Verification items for the finished model (mm, model axes). Face numbers are marked on the shaded views. Coordinates: 2 decimals unless noted, no trailing zeros. Order: outer loops, then holes, each group sorted by start corner. A loop starts at its lowest first (then second) coordinate and runs counter-clockwise, first axis right, second up. Notation, with made-up numbers: M 78,-35.5 L 92,-35.5 A14 cw 92,-30.5 Z; hole C 40,62.25 d7. An arc over 180 degrees is marked long. Answer as a JSON object with one key per item and string values. Group by question number.
(1) Gauge pin test, flat ends, axial feed: pin 1 Ø1 at (y, z) = (29, 10) entering from +X; pin 2 Ø4 at (y, z) = (17, 13.5) entering from +X; pin 3 Ø1.5 at (y, z) = (36.5, 12.5) entering from +X. Record the tip position at first contact, or that the pin passes through.
(2) Cross-section at A-A (x = 18). Enter the section's corners in (y, z).
(3) Material ranges on line 1 (X direction, y = 33.75, z = 8.5); line 2 (X direction, y = 16, z = 10); line 3 (X direction, y = 27, z = 11.5), recorded low to high.
(4) Cross-section at B-B (y = 24.75). Enter the section's corners in (x, z), plus the area to 3 significant figures.
(5) Cross-section at C-C (z = 10). Enter the section's corners in (x, y).
(6) Cross-section at D-D (x = -55.5). Enter the section's corners in (y, z).
(7) Mould release check, pull along Y, two halves, no side actions. Record for the marked faces 1, 2, 3 and 4: released by +Y, released by -Y, zero draft, split by the parting line, or undercut.
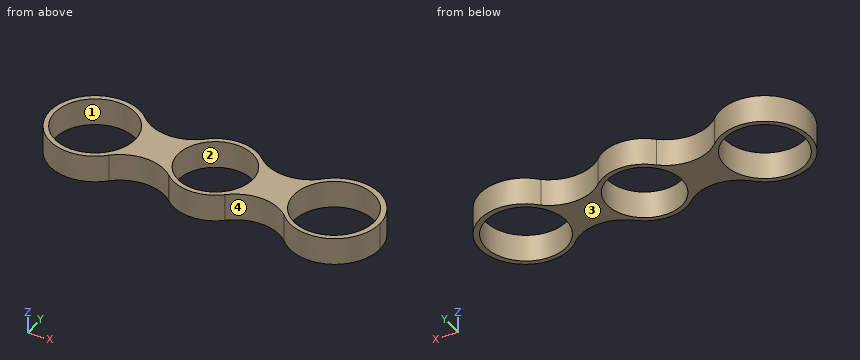
from build123d import *

# Parameters (mm, degrees)
F1_DEPTH = 8
F3_DEPTH = 8
F4_D     = 23.6
F5_D     = 22


# Not quite as in the source:
# - a feature names something its author has since deleted; it is built from what else it names


with BuildPart() as f1:
    # F0 (on Top) → F1 (new body)
    with BuildSketch(Plane.XY):
        with BuildLine():
            ThreePointArc((30.2364596242, 25.5677551031), (18.556965651, 37.3204786398), (6.7314716859, 25.7146705041))
            ThreePointArc((6.7314716859, 25.7146705041), (18.4100473802, 13.8150315665), (30.2364596242, 25.5677551031))
        make_face()
    extrude(amount=F1_DEPTH)

    # F2 (on face) → F3 (join)
    with BuildSketch(Plane.XY.offset(8)):
        with BuildLine():
            ThreePointArc((-42.5114348153, 35.1915450581), (-65.2620832709, 26.0556201481), (-42.5726949965, 16.7685975444))
            ThreePointArc((-42.5726949965, 16.7685975444), (-39.7847972392, 21.021355147), (-38.8073447634, 26.0116364807))
            ThreePointArc((-38.8073447634, 26.0116364807), (-39.7682713179, 30.9611567757), (-42.5114348153, 35.1915450581))
        make_face()
        with BuildLine():
            ThreePointArc((-38.8073447634, 26.0116364807), (-39.7847972392, 21.021355147), (-42.5726949965, 16.7685975444))
            ThreePointArc((-42.5726949965, 16.7685975444), (-33.87370444, 20.218317429), (-25.1016516698, 16.9588551759))
            ThreePointArc((-25.1016516698, 16.9588551759), (-29.0338445102, 25.8480071098), (-25.3315074449, 34.8353238892))
            ThreePointArc((-25.3315074449, 34.8353238892), (-33.9883630197, 31.7873549926), (-42.5114348153, 35.1915450581))
            ThreePointArc((-42.5114348153, 35.1915450581), (-39.7682713179, 30.9611567757), (-38.8073447634, 26.0116364807))
        make_face()
        with BuildLine():
            ThreePointArc((-24.8354704192, 16.7176675443), (-24.9677312973, 16.8391770918), (-25.1016516698, 16.9588551759))
            ThreePointArc((-25.1016516698, 16.9588551759), (-24.9694362403, 16.8372954701), (-24.8354704192, 16.7176675443))
        make_face()
        with BuildLine():
            ThreePointArc((-25.3315074449, 34.8353238892), (-29.0338445102, 25.8480071098), (-25.1016516698, 16.9588551759))
            ThreePointArc((-25.1016516698, 16.9588551759), (-24.9677312973, 16.8391770918), (-24.8354704192, 16.7176675443))
            ThreePointArc((-24.8354704192, 16.7176675443), (-16.6524528686, 13.6328843719), (-8.4735280262, 16.7285025458))
            ThreePointArc((-8.4735280262, 16.7285025458), (-8.4359829057, 16.7620336333), (-8.3983087423, 16.7954196681))
            ThreePointArc((-8.3983087423, 16.7954196681), (-5.3610604956, 20.9632278118), (-4.2864270488, 26.0071017784))
            ThreePointArc((-4.2864270488, 26.0071017784), (-5.2792843636, 30.8636339026), (-8.098530607, 34.9408290832))
            ThreePointArc((-8.098530607, 34.9408290832), (-16.7364042498, 38.381089997), (-25.3315074449, 34.8353238892))
        make_face()
        with BuildLine():
            ThreePointArc((8.8624930635, 34.5276918287), (0.3063045577, 31.6274145181), (-8.098530607, 34.9408290832))
            ThreePointArc((-8.098530607, 34.9408290832), (-5.2792843636, 30.8636339026), (-4.2864270488, 26.0071017784))
            ThreePointArc((-4.2864270488, 26.0071017784), (-5.3610604956, 20.9632278118), (-8.3983087423, 16.7954196681))
            ThreePointArc((-8.3983087423, 16.7954196681), (0.2487240262, 20.0624034029), (8.8910160496, 16.7828993238))
            ThreePointArc((8.8910160496, 16.7828993238), (5.4597887201, 25.6498031441), (8.8624930635, 34.5276918287))
        make_face()
        with BuildLine():
            ThreePointArc((-8.3983087423, 16.7954196681), (-8.4359829057, 16.7620336333), (-8.4735280262, 16.7285025458))
            ThreePointArc((-8.4735280262, 16.7285025458), (-8.4358503291, 16.7618846084), (-8.3983087423, 16.7954196681))
        make_face()
        with BuildLine():
            ThreePointArc((31.9145832669, 25.6710648537), (23.431077599, 38.0185211111), (8.8624930635, 34.5276918287))
            ThreePointArc((8.8624930635, 34.5276918287), (5.4597887201, 25.6498031441), (8.8910160496, 16.7828993238))
            ThreePointArc((8.8910160496, 16.7828993238), (23.4509187507, 13.3312498845), (31.9145832669, 25.6710648537))
        make_face()
    extrude(amount=F3_DEPTH)

    # F4 (through all)
    with Locations(Plane(origin=(0, 0, 0), x_dir=(1, 0, 0), z_dir=(0, 0, -1))):
        with Locations((-52.0347505808, -26.0116364807), (18.4835065156, -25.5677551031)):
            Hole(F4_D / 2)

    # F5 (through all)
    with Locations(Plane(origin=(0, 0, 0), x_dir=(1, 0, 0), z_dir=(0, 0, -1))):
        with Locations((-16.6606471685, -26.0071017784)):
            Hole(F5_D / 2)


solid = f1.part
Taken from the geometry:
{
 "1": {"pin 1": "stops at x = 31.61", "pin 2": "stops at x = 30.11", "pin 3": "stops at x = 27.25"},
 "2": {"outline": "M 12.46,8 L 13.78,8 L 13.78,16 L 12.46,16 Z; M 37.36,8 L 38.88,8 L 38.88,16 L 37.36,16 Z"},
 "3": {"line 1": "x = -62.76 to -60.94, -43.13 to -40.61, -26.83 to -24.47, -8.85 to -6.54, 7.79 to 9.98, 26.99 to 29.16", "line 2": "x = -60.68 to -58.28, -45.79 to -43.39, -23.94 to -21.23, -12.09 to -9.38, 9.66 to 11.58, 25.39 to 27.71", "line 3": "x = -65.23 to -63.79, -40.28 to -27.62, -5.71 to 6.77, 30.2 to 31.85"},
 "4": {"outline": "M -65.2,8 L -63.77,8 L -63.77,16 L -65.2,16 Z; M -40.3,8 L -27.59,8 L -27.59,16 L -40.3,16 Z; M -5.73,8 L 6.71,8 L 6.71,16 L -5.73,16 Z; M 30.26,8 L 31.88,8 L 31.88,16 L 30.26,16 Z", "area": "226 mm²"},
 "5": {"outline": "M -42.57,16.77 A13.05 cw -25.1,16.96 A12.37 ccw -8.4,16.8 A13.05 cw 8.89,16.78 A13.23 ccw long 8.86,34.53 A13.13 cw -8.1,34.94 A12.37 ccw -25.33,34.84 A13.05 cw -42.51,35.19 A13.23 ccw long Z; hole C -52.03,26.01 d23.6; hole C -16.66,26.01 d22; hole C 18.48,25.57 d23.6"},
 "6": {"outline": "M 13.25,8 L 14.73,8 L 14.73,16 L 13.25,16 Z; M 37.29,8 L 38.78,8 L 38.78,16 L 37.29,16 Z"},
 "7": {"face 1": "undercut", "face 2": "undercut", "face 3": "zero draft", "face 4": "released by -Y"}
}
